The model under review builds one solid part; all positions refer to its coordinate system, in mm. Give positions to 0.01 mm unless a question says otherwise; leave off trailing zeros. Loops run counter-clockwise (first coordinate to the right, second up) from the corner with the lowest first, then second, coordinate; pieces in that order, holes last. Notation, with made-up numbers: M -20,12 L 9,12 A26 ccw 9,43 Z; hole C 34,1.25 d9. An arc over 180 degrees is marked long. Put each result on its own line as item: value. Start each with the question number.
```python
from build123d import *

# Parameters (mm, degrees)
SCHIZZO1_W                      = 160
SCHIZZO1_H                      = 150
BASE_DEPTH                      = 3
SCHIZZO2_W                      = 10
SCHIZZO2_H                      = 68
TAGLIOPMSINISTRA_DEPTH          = 110.69958979
SCHIZZO6_W                      = 45
SCHIZZO6_H                      = 3.5
FOROBECBASSO_DEPTH              = 110.69958979
SCHIZZO8_R                      = 1.5
FORIVITIPM_DEPTH                = 110.69958979
SCHIZZO9_R                      = 1.5
FORIVITICOMPANION_DEPTH         = 110.69958979
SCHIZZO12_R                     = 1.75
FORICOLLEGAMENTOFUSOLIERA_DEPTH = 110.69958979
SCHIZZO13_W                     = 10
SCHIZZO13_H                     = 68
CHIUSURATAGLIOSINISTROPM_DEPTH  = 3


with BuildPart() as part:
    # Schizzo1 → Base (new body)
    with BuildSketch(Plane(origin=(0, 0, 0), x_dir=(1, 0, 0), z_dir=(0, 1, 0))):
        Rectangle(SCHIZZO1_W, SCHIZZO1_H)
    extrude(amount=BASE_DEPTH)

    # Schizzo2 → TaglioPMSinistra (cut, through all)
    with BuildSketch(Plane(origin=(0, 3, 0), x_dir=(1, 0, 0), z_dir=(0, 1, 0))):
        with Locations((-58, -38)):
            Rectangle(SCHIZZO2_W, SCHIZZO2_H)
    tagliopmsinistra = extrude(amount=-TAGLIOPMSINISTRA_DEPTH, mode=Mode.SUBTRACT)

    # TaglioPMDestra: TaglioPMSinistra across plane
    add(tagliopmsinistra.mirror(Plane(origin=(-23, 0, 0), x_dir=(0, 0, 1), z_dir=(1, 0, 0))), mode=Mode.SUBTRACT)

    # Schizzo6 → ForoBECBasso (cut, through all)
    with BuildSketch(Plane(origin=(0, 3, 0), x_dir=(1, 0, 0), z_dir=(0, 1, 0))):
        with Locations((45.5, -68.25)):
            Rectangle(SCHIZZO6_W, SCHIZZO6_H)
    forobecbasso = extrude(amount=-FOROBECBASSO_DEPTH, mode=Mode.SUBTRACT)

    # ForoBECAlto: ForoBECBasso across plane
    add(forobecbasso.mirror(Plane.XY.offset(52.5)), mode=Mode.SUBTRACT)

    # Schizzo8 → ForiVitiPM (cut, through all)
    with BuildSketch(Plane(origin=(0, 3, 0), x_dir=(1, 0, 0), z_dir=(0, 1, 0))):
        with Locations(Location((-70.5, -3, 0), (0, 0, 270))):
            Circle(SCHIZZO8_R)
        with Locations(Location((-70.5, -48, 0), (0, 0, 270))):
            Circle(SCHIZZO8_R)
        with Locations(Location((-25.5, -48, 0), (0, 0, 90))):
            Circle(SCHIZZO8_R)
        with Locations(Location((-25.5, -3, 0), (0, 0, 90))):
            Circle(SCHIZZO8_R)
    extrude(amount=-FORIVITIPM_DEPTH, mode=Mode.SUBTRACT)

    # Schizzo9 → ForiVitiCompanion (cut, through all)
    with BuildSketch(Plane(origin=(0, 3, 0), x_dir=(1, 0, 0), z_dir=(0, 1, 0))):
        with Locations(Location((60.7, -27.7, 0), (0, 0, 270))):
            Circle(SCHIZZO9_R)
        with Locations(Location((25.3, -27.7, 0), (0, 0, 270))):
            Circle(SCHIZZO9_R)
        with Locations(Location((25.3, 7.7, 0), (0, 0, 270))):
            Circle(SCHIZZO9_R)
        with Locations(Location((60.7, 7.7, 0), (0, 0, 270))):
            Circle(SCHIZZO9_R)
    extrude(amount=-FORIVITICOMPANION_DEPTH, mode=Mode.SUBTRACT)

    # Schizzo12 → ForiCollegamentoFusoliera (cut, through all)
    with BuildSketch(Plane(origin=(0, 3, 0), x_dir=(1, 0, 0), z_dir=(0, 1, 0))):
        with Locations(Location((-75, 70, 0), (0, 0, 270))):
            Circle(SCHIZZO12_R)
        with Locations(Location((75, 70, 0), (0, 0, 270))):
            Circle(SCHIZZO12_R)
        with Locations(Location((0, 70, 0), (0, 0, 270))):
            Circle(SCHIZZO12_R)
        with Locations(Location((-75, -70, 0), (0, 0, 270))):
            Circle(SCHIZZO12_R)
        with Locations(Location((0, -70, 0), (0, 0, 270))):
            Circle(SCHIZZO12_R)
        with Locations(Location((75, -70, 0), (0, 0, 270))):
            Circle(SCHIZZO12_R)
    extrude(amount=-FORICOLLEGAMENTOFUSOLIERA_DEPTH, mode=Mode.SUBTRACT)

    # Schizzo13 → ChiusuraTaglioSinistroPM (add, through all)
    with BuildSketch(Plane(origin=(0, 3, 0), x_dir=(1, 0, 0), z_dir=(0, 1, 0))):
        with Locations((-58, -38)):
            Rectangle(SCHIZZO13_W, SCHIZZO13_H)
    extrude(amount=-CHIUSURATAGLIOSINISTROPM_DEPTH)


solid = part.part
```
Item 1: Consider section A-A, the plane z = 19. Write out the cut boundary in (x, y).
Item 2: Consider section C-C, the plane x = 37.5. Write out the cut boundary in (y, z).
Item 3: Draft analysis for pull direction Z (two halves, no side actions). For faces 1 (the cylindrical face through (0.526, 1.521, -68.331)), 2 (the flat face through (-1, 0, -1)), state which applies: +Z half, -Z half, draft (parallel to the pull), parting line (faces both ways), or undercut.
Item 4: To check wall thickness, follow L1, parallel to Z at x = 65, y = 1.2; L2, parallel to X at y = 1.65, z = 27.7; L3, parallel to X at y = 1.5, z = 48. State the ranges of each line that lie inside material, in increasing order. Write a range as [from, to].
Item 5: Consider section B-B, the plane y = 1.1. Give the number of separate pieces and of enclosed holes in the cut face, plus the area to 3 significant figures.
Report:
1. outline: M -80,0 L 7,0 L 7,3 L -80,3 Z; M 17,0 L 80,0 L 80,3 L 17,3 Z
2. outline: M 0,-75 L 3,-75 L 3,35 L 0,35 Z; M 0,38.5 L 3,38.5 L 3,66.5 L 0,66.5 Z; M 0,70 L 3,70 L 3,75 L 0,75 Z
3. face 1: undercut
3. face 2: draft
4. L1: [-75, 35], [38.5, 66.5], [70, 75]
4. L2: [-80, 7], [17, 23.8], [26.8, 59.2], [62.2, 80]
4. L3: [-80, -72], [-69, -27], [-24, 7], [17, 80]
5. separate pieces: 1
5. enclosed holes: 17
5. area: 22,900 mm²
